The listing builds one solid part. Answer for the finished solid, in the listing's coordinates (mm). Coordinates: 2 decimals unless noted, no trailing zeros. Order: outer loops, then holes, each group sorted by start corner. A loop starts at its lowest first (then second) coordinate and runs counter-clockwise, first axis right, second up. Notation, with made-up numbers: (32.5, 33) -> (54.5, 33) arc R34 cw to (54.5, 64) -> close; hole circle Ø4 at (-13.75, 33.25). An arc over 180 degrees is marked (long way). Answer in a Markdown table with one row per item.
```python
from build123d import *

# Parameters (mm, degrees)
SKETCH1_W           = 284
SKETCH1_H           = 71
BOSS_EXTRUDE1_DEPTH = 2
BOSS_EXTRUDE2_DEPTH = 0.5


with BuildPart() as part:
    # Sketch1 → Boss-Extrude1 (new body)
    with BuildSketch(Plane.XY):
        with Locations((-0.375320298, 122.74793824)):
            Rectangle(SKETCH1_W, SKETCH1_H)
        Polygon((122.049253222, 148.94793824), (123.636966462, 146.19793824), (126.812392942, 146.19793824), (128.400106183, 148.94793824), (126.812392942, 151.69793824), (123.636966462, 151.69793824), align=None, mode=Mode.SUBTRACT)
        Polygon((122.049253222, 98.04793824), (123.636966462, 95.29793824), (126.812392942, 95.29793824), (128.400106183, 98.04793824), (126.812392942, 100.79793824), (123.636966462, 100.79793824), align=None, mode=Mode.SUBTRACT)
        Polygon((-131.980746778, 98.04793824), (-130.393033538, 95.29793824), (-127.217607058, 95.29793824), (-125.629893817, 98.04793824), (-127.217607058, 100.79793824), (-130.393033538, 100.79793824), align=None, mode=Mode.SUBTRACT)
        Polygon((-125.629893817, 148.94793824), (-127.217607058, 151.69793824), (-130.393033538, 151.69793824), (-131.980746778, 148.94793824), (-130.393033538, 146.19793824), (-127.217607058, 146.19793824), align=None, mode=Mode.SUBTRACT)
        Polygon((-61.050746778, 98.04793824), (-59.463033538, 95.29793824), (-56.287607058, 95.29793824), (-54.699893817, 98.04793824), (-56.287607058, 100.79793824), (-59.463033538, 100.79793824), align=None, mode=Mode.SUBTRACT)
        Polygon((-61.050746778, 148.94793824), (-59.463033538, 146.19793824), (-56.287607058, 146.19793824), (-54.699893817, 148.94793824), (-56.287607058, 151.69793824), (-59.463033538, 151.69793824), align=None, mode=Mode.SUBTRACT)
        Polygon((61.049253222, 148.94793824), (62.636966462, 146.19793824), (65.812392942, 146.19793824), (67.400106183, 148.94793824), (65.812392942, 151.69793824), (62.636966462, 151.69793824), align=None, mode=Mode.SUBTRACT)
        Polygon((61.049253222, 98.04793824), (62.636966462, 95.29793824), (65.812392942, 95.29793824), (67.400106183, 98.04793824), (65.812392942, 100.79793824), (62.636966462, 100.79793824), align=None, mode=Mode.SUBTRACT)
    extrude(amount=BOSS_EXTRUDE1_DEPTH)

    # Sketch2 → Boss-Extrude2 (add)
    with BuildSketch(Plane.XY.offset(2)):
        Polygon((-113.14842838, 140.954026683), (-113.14842838, 144.897894949), (-114.711093164, 144.897894949), (-112.106651856, 148.172049737), (-110.246336636, 144.897894949), (-111.176494246, 144.897894949), (-111.176494246, 140.954026683), align=None)
    extrude(amount=BOSS_EXTRUDE2_DEPTH)


solid = part.part
```
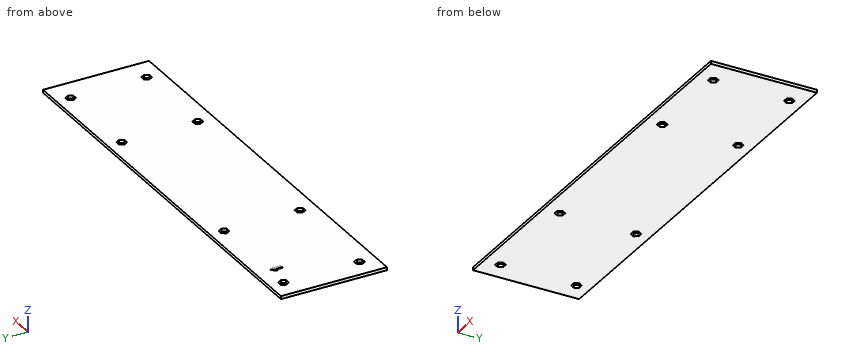
(1) A cutting plane is placed at B-B, the plane y = 105. Determine the outline of the cut face in (x, z).
Check values:
| item | result |
|---|---|
| outline | (-142.38, 0) -> (141.62, 0) -> (141.62, 2) -> (-142.38, 2) -> close |
(2) A cutting plane is placed at A-A, the plane x = 97. Determine the outline of the cut face in (y, z).
Check values:
| item | result |
|---|---|
| outline | (87.25, 0) -> (158.25, 0) -> (158.25, 2) -> (87.25, 2) -> close |
(3) Flat-ended cylindrical pins translate along their axes: pin 1 (10 mm diameter, centred on x = -15, y = 111, fed in from -Z); pin 2 (1 mm diameter, centred on x = -91, y = 123, fed in from +Z). Find the tip coordinate at first contact, or state that the pin passes through.
Check values:
| item | result |
|---|---|
| pin 1 | z = 0 |
| pin 2 | z = 2 |
(4) Find the intervals of material crossed by line 1 along Y through (x, z) = (-128, 0.2); line 2 along Z through (x, y) = (79.5, 114.5); line 3 along X through (y, z) = (99.5, 1), in increasing order. Write a range as from..to.
Check values:
| item | result |
|---|---|
| line 1 | 87.25..95.3, 100.8..146.2, 151.7..158.25 |
| line 2 | 0..2 |
| line 3 | -142.38..-131.14, -126.47..-60.21, -55.54..61.89, 66.56..122.89, 127.56..141.62 |
